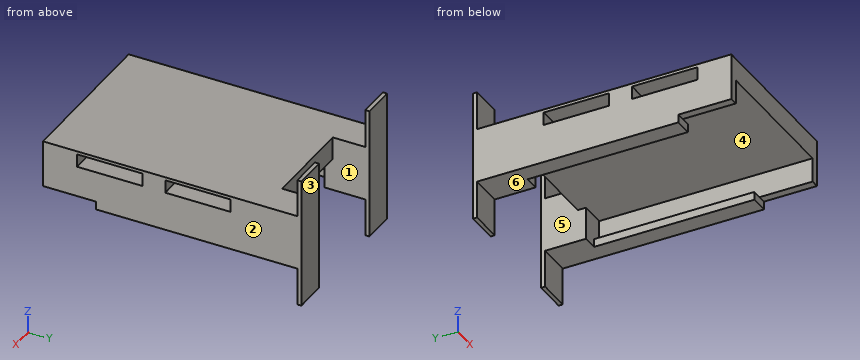
from build123d import *

# Parameters (mm, degrees)
BOSS_EXTRUDE1_DEPTH = 83.0326
SKETCH6_W           = 61.8998
SKETCH6_H           = 21.463
BOSS_EXTRUDE3_DEPTH = 3.175
SKETCH7_W           = 16.5354
SKETCH7_H           = 9.525
CUT_EXTRUDE2_DEPTH  = 91.420129415
SKETCH8_W           = 5.08
SKETCH8_H           = 25.4
CUT_EXTRUDE3_DEPTH  = 108.64212172
SKETCH15_W          = 61.8998
SKETCH15_H          = 20.63242
CUT_EXTRUDE4_DEPTH  = 3.175
SKETCH16_W          = 36.4998
SKETCH16_H          = 12.7
CUT_EXTRUDE5_DEPTH  = 3.175
SKETCH17_W          = 12.7
SKETCH17_H          = 21.463
BOSS_EXTRUDE4_DEPTH = 12.7
SKETCH18_W          = 12.7
SKETCH18_H          = 50.8
BOSS_EXTRUDE5_DEPTH = 1.5875
SKETCH19_W          = 12.7
SKETCH19_H          = 51.208048645
BOSS_EXTRUDE6_DEPTH = 1.5875


with BuildPart() as part:
    # Sketch1 → Boss-Extrude1 (new body)
    with BuildSketch(Plane(origin=(0, 0, 0), x_dir=(1, 0, 0), z_dir=(0, 1, 0))):
        Polygon((-30.9499, -3.477149156), (30.9499, -3.477149156), (30.9499, 17.985850844), (24.0411, 17.985850844), (24.0411, 14.810850844), (27.7749, 14.810850844), (27.7749, 5.285850844), (-27.7749, 5.285850844), (-27.7749, 14.810850844), (-24.0411, 14.810850844), (-24.0411, 17.985850844), (-30.9499, 17.985850844), align=None)
    extrude(amount=BOSS_EXTRUDE1_DEPTH)

    # Sketch6 → Boss-Extrude3 (add)
    with BuildSketch(Plane(origin=(0, 83.0326, 0), x_dir=(1, 0, 0), z_dir=(0, 1, 0))):
        with Locations((0, 7.254350844)):
            Rectangle(SKETCH6_W, SKETCH6_H)
    extrude(amount=BOSS_EXTRUDE3_DEPTH)

    # Sketch7 → Cut-Extrude2 (cut, through all)
    with BuildSketch(Plane.XZ.offset(-83.0326)):
        with Locations((0, -10.048350844)):
            Rectangle(SKETCH7_W, SKETCH7_H)
    extrude(amount=-CUT_EXTRUDE2_DEPTH, mode=Mode.SUBTRACT)

    # Sketch8 → Cut-Extrude3 (cut, through all)
    with BuildSketch(Plane.ZY.offset(30.9499)):
        with Locations((-0.274453158, 60.28364576)):
            Rectangle(SKETCH8_W, SKETCH8_H)
        with Locations((-0.274453158, 25.92395424)):
            Rectangle(SKETCH8_W, SKETCH8_H)
    extrude(amount=-CUT_EXTRUDE3_DEPTH, mode=Mode.SUBTRACT)

    # Sketch15 → Cut-Extrude4 (cut)
    with BuildSketch(Plane(origin=(0, 0, -17.985850844), x_dir=(-1, 0, 0), z_dir=(0, 0, -1))):
        with Locations((0, 10.31621)):
            Rectangle(SKETCH15_W, SKETCH15_H)
    extrude(amount=-CUT_EXTRUDE4_DEPTH, mode=Mode.SUBTRACT)

    # Sketch16 → Cut-Extrude5 (cut)
    with BuildSketch(Plane(origin=(0, 86.2076, 0), x_dir=(1, 0, 0), z_dir=(0, 1, 0))):
        with Locations((0, 11.635850844)):
            Rectangle(SKETCH16_W, SKETCH16_H)
    extrude(amount=-CUT_EXTRUDE5_DEPTH, mode=Mode.SUBTRACT)

    # Sketch17 → Boss-Extrude4 (add)
    with BuildSketch(Plane(origin=(0, 86.2076, 0), x_dir=(1, 0, 0), z_dir=(0, 1, 0))):
        with Locations((-24.5999, 7.254350844)):
            Rectangle(SKETCH17_W, SKETCH17_H)
        with Locations((24.5999, 7.254350844)):
            Rectangle(SKETCH17_W, SKETCH17_H)
    extrude(amount=BOSS_EXTRUDE4_DEPTH)

    # Sketch18 → Boss-Extrude5 (add)
    with BuildSketch(Plane(origin=(0, 98.9076, 0), x_dir=(1, 0, 0), z_dir=(0, 1, 0))):
        with Locations((24.5999, 7.254350844)):
            Rectangle(SKETCH18_W, SKETCH18_H)
    extrude(amount=BOSS_EXTRUDE5_DEPTH)

    # Sketch19 → Boss-Extrude6 (add)
    with BuildSketch(Plane(origin=(0, 98.9076, 0), x_dir=(1, 0, 0), z_dir=(0, 1, 0))):
        with Locations((-24.5999, 7.050326521)):
            Rectangle(SKETCH19_W, SKETCH19_H)
    extrude(amount=BOSS_EXTRUDE6_DEPTH)


solid = part.part
Verification items for the finished model (mm, model axes). Face numbers are marked on the shaded views. A direction names the side the tool comes from. Coordinates: 2 decimals unless noted, no trailing zeros. Order: outer loops, then holes, each group sorted by start corner. A loop starts at its lowest first (then second) coordinate and runs counter-clockwise, first axis right, second up. Notation, with made-up numbers: M -31,23 L -4,23 A31 ccw -4,53 Z; hole C -25.5,17 d4. An arc over 180 degrees is marked long. One line per item, written item: value. Start each with the question number.
Item 1: Sectioned sample at A-A on z = 15.5. Record the cut outline in (x, y), then the cut area to 3 significant figures.
Item 2: Mould release check, pull along X, two halves, no side actions. Record for the marked faces 1, 2 and 3: pulls with the +X half, pulls with the -X half, needs draft (parallel to the pull), parting line crosses it, or undercut.
Item 3: Sectioned sample at D-D on y = 7. Record the cut outline in (x, z), then the cut area to 3 significant figures.
Item 4: Access from +Z, -Z, +X, -X, +Y, -Y to the whole of each face (thin tool, end or side, straight path). Record for the marked faces 4, 5 and 6.
Item 5: Sectioned sample at C-C on x = -9.5. Record the cut outline in (y, z).
Item 6: Sectioned sample at B-B on y = 57.5. Record the cut outline in (x, z).
Item 7: Thickness scan on probe 1 along Y at (x, z) = (2, 0); probe 2 along Z at (x, y) = (26, 26); probe 3 along Z at (x, y) = (-18.5, 33.5). Record the ranges inside material, lowest first.
Item 8: Depth check by flat-ended pin: P1, Ø4, axis at x = -25, y = 39, coming from the +Z side; P2, Ø4, axis at x = -13, z = 0.5, coming from the +Y side; P3, Ø4, axis at x = 22.5, y = 44.5, coming from the -Z side. Enter the tip coordinate at first touch or a pass-through.
Calculated:
1. outline: M -30.95,98.91 L -18.25,98.91 L -18.25,100.5 L -30.95,100.5 Z; M 18.25,98.91 L 30.95,98.91 L 30.95,100.5 L 18.25,100.5 Z
1. area: 40.3 mm^2
2. face 1: undercut
2. face 2: pulls with the +X half
2. face 3: needs draft
3. outline: M -30.95,-14.81 L -27.77,-14.81 L -27.77,-5.29 L 27.77,-5.29 L 27.77,-14.81 L 30.95,-14.81 L 30.95,3.48 L -30.95,3.48 Z
3. area: 603 mm^2
4. face 4: -Y
4. face 5: -Z, +Y
4. face 6: -Z, +X, -X, -Y
5. outline: M 0,-5.29 L 86.21,-5.29 L 86.21,3.48 L 0,3.48 Z; hole M 13.22,-2.81 L 38.62,-2.81 L 38.62,2.27 L 13.22,2.27 Z; hole M 47.58,-2.81 L 72.98,-2.81 L 72.98,2.27 L 47.58,2.27 Z
6. outline: M -30.95,-17.99 L -24.04,-17.99 L -24.04,-14.81 L -27.77,-14.81 L -27.77,-5.29 L 27.77,-5.29 L 27.77,-14.81 L 24.04,-14.81 L 24.04,-17.99 L 30.95,-17.99 L 30.95,-2.81 L -30.95,-2.81 Z; M -30.95,2.27 L 30.95,2.27 L 30.95,3.48 L -30.95,3.48 Z
7. probe 1: 0 to 13.22, 38.62 to 47.58, 72.98 to 86.21
7. probe 2: -17.99 to -14.81, -5.29 to -2.81, 2.27 to 3.48
7. probe 3: -5.29 to -2.81, 2.27 to 3.48
8. P1: z = 3.48
8. P2: y = 86.21
8. P3: z = -17.99
